```python
from build123d import *

# Parameters (mm, degrees)
BOSS_EXTRUDE1_DEPTH = 5.63
FILLET1_R           = 28
SKETCH2_R           = 4
CUT_EXTRUDE4_DEPTH  = 10


with BuildPart() as part:
    # Sketch1 → Boss-Extrude1 (new body)
    with BuildSketch(Plane(origin=(0, 0, 0), x_dir=(1, 0, 0), z_dir=(0, 1, 0))):
        Polygon((-7.5, 147.657331345), (-85.25, 147.657331345), (-170.5, 0), (-131.650528172, -67.289259053), (-134.205303113, -68.764259053), (-126.705303113, -81.75464011), (-124.150528172, -80.27964011), (-85.25, -147.657331345), (0, -295.31466269), (85.25, -147.657331345), (124.150528172, -80.27964011), (126.705303113, -81.75464011), (134.205303113, -68.764259053), (131.650528172, -67.289259053), (170.5, 0), (85.25, 147.657331345), (7.5, 147.657331345), (7.5, 150.607331345), (-7.5, 150.607331345), align=None)
    extrude(amount=BOSS_EXTRUDE1_DEPTH)

    # Fillet1
    fillet1_edges = [part.edges().sort_by_distance(p)[0] for p in [
        (0, 2.815, 295.31466269),
    ]]
    fillet(fillet1_edges, radius=FILLET1_R)

    # Sketch2 → Cut-Extrude4 (cut)
    with BuildSketch(Plane(origin=(0, 5.63, 0), x_dir=(1, 0, 0), z_dir=(0, 1, 0))):
        with Locations(Location((0, -251.834791554, 0), (0, 0, 270))):
            Circle(SKETCH2_R)
    extrude(amount=-CUT_EXTRUDE4_DEPTH, mode=Mode.SUBTRACT)


solid = part.part
```
The listing builds one solid part. Answer for the finished solid, in the listing's coordinates (mm). Give positions to 0.01 mm unless a question says otherwise; leave off trailing zeros. Loops run counter-clockwise (first coordinate to the right, second up) from the corner with the lowest first, then second, coordinate; pieces in that order, holes last. Notation, with made-up numbers: (-34.5, -19.75) - (23.5, -19.75) arc R13 cw to (23.5, -5.75) - close; hole circle Ø4 at (60, 69). An arc over 180 degrees is marked (long way). Return JSON: item names as keys, results as strings. Group by question number.
1. Straight lines are drawn through the part: line 1 (X direction, y = 2.05, z = 12); line 2 (X direction, y = 2.9, z = 172.5); line 3 (Z direction, x = -96, y = 1.35). For each, find the intervals that lie inside material, in ascending order. Write a range as [from, to].
2. Find section C-C (z = 182). Write down the section's boundary in (x, y), then the cut area to 3 significant figures.
3. Find section A-A (y = 1.15). Write down the section's boundary in (x, z), then the cut area to 3 significant figures.
4. Find section B-B (x = 103). Write down the section's boundary in (y, z), then the cut area to 3 significant figures.
5. Given pin 1 Ø1 at (y, z) = (4.5, 181.5) entering from +X; pin 2 Ø3 at (y, z) = (1.5, -149.5) entering from +X; pin 3 Ø5 at (x, z) = (41.5, 201) entering from -Y; pin 4 Ø0.9 at (y, z) = (4, -149) entering from -X, each flat-ended and moving along its own axis, determine where each tip first touches the part or whether it passes through.
Verdict:
{
 "1": {"line 1": "x = [-163.57, 163.57]", "line 2": "x = [-70.91, 70.91]", "line 3": "z = [-129.04, 129.04]"},
 "2": {"outline": "(-65.42, 0) - (65.42, 0) - (65.42, 5.63) - (-65.42, 5.63) - close", "area": "737 mm^2"},
 "3": {"outline": "(-170.5, 0) - (-85.25, -147.66) - (-7.5, -147.66) - (-7.5, -150.61) - (7.5, -150.61) - (7.5, -147.66) - (85.25, -147.66) - (170.5, 0) - (131.65, 67.29) - (134.21, 68.76) - (126.71, 81.75) - (124.15, 80.28) - (24.25, 253.31) arc R28 ccw to (-24.25, 253.31) - (-124.15, 80.28) - (-126.71, 81.75) - (-134.21, 68.76) - (-131.65, 67.29) - close; hole circle Ø8 at (0, 251.83)", "area": "87,700 mm^2"},
 "4": {"outline": "(0, -116.91) - (5.63, -116.91) - (5.63, 116.91) - (0, 116.91) - close", "area": "1,320 mm^2"},
 "5": {"pin 1": "stops at x = 66", "pin 2": "stops at x = 7.5", "pin 3": "stops at y = 0", "pin 4": "stops at x = -7.5"}
}
